from build123d import *

# Parameters (mm, degrees)
SKETCH1_W           = 86.36
SKETCH1_H           = 76.2
SKETCH1_R           = 1.397
BOSS_EXTRUDE1_DEPTH = 2
SKETCH2_W           = 15.24
SKETCH2_H           = 2.54
BOSS_EXTRUDE2_DEPTH = 40


with BuildPart() as part:
    # Sketch1 → Boss-Extrude1 (new body)
    with BuildSketch(Plane(origin=(0, 0, 0), x_dir=(1, 0, 0), z_dir=(0, 1, 0))):
        Rectangle(SKETCH1_W, SKETCH1_H)
        with Locations((-39.37, 34.29)):
            Circle(SKETCH1_R, mode=Mode.SUBTRACT)
        with Locations((39.37, -34.29)):
            Circle(SKETCH1_R, mode=Mode.SUBTRACT)
        with Locations((-39.37, -34.29)):
            Circle(SKETCH1_R, mode=Mode.SUBTRACT)
        with Locations((39.37, 34.29)):
            Circle(SKETCH1_R, mode=Mode.SUBTRACT)
    extrude(amount=BOSS_EXTRUDE1_DEPTH)

    # Sketch2 → Boss-Extrude2 (add)
    with BuildSketch(Plane(origin=(0, 2, 0), x_dir=(1, 0, 0), z_dir=(0, 1, 0))):
        with Locations((-16.51, 2.54)):
            Rectangle(SKETCH2_W, SKETCH2_H)
    extrude(amount=BOSS_EXTRUDE2_DEPTH)


solid = part.part
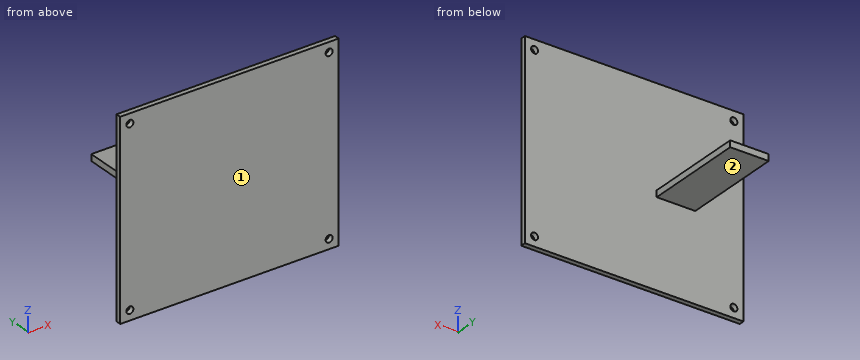
Check sheet for the modelled part. Datum: model origin and axes. Units: mm. Face numbers are marked on the shaded views. A direction names the side the tool comes from. Coordinates: 2 decimals unless noted, no trailing zeros. Loops run counter-clockwise (first coordinate to the right, second up) from the corner with the lowest first, then second, coordinate; pieces in that order, holes last. Notation, with made-up numbers: (-34, 52.5) -> (17, 52.5) arc R27 cw to (17, 86.5) -> close; hole circle Ø6 at (57, 51.25). An arc over 180 degrees is marked (long way). Write item = value, one per line. Start each with the question number.
1. Depth check by flat-ended pin: P1, Ø7.5, axis at x = -19, y = 18.5, coming from the -Z side; P2, Ø1.7, axis at x = -39.37, z = 34.29, coming from the +Y side; P3, Ø3, axis at x = 20, z = -18, coming from the +Y side; P4, Ø12, axis at x = -16, y = 26.5, coming from the +Z side. Enter the tip coordinate at first touch or a pass-through.
2. Section check D-D on y = 33. Record the cut outline in (x, z).
3. Section check C-C on x = -16. Record the cut outline in (y, z), then the cut area to 3 significant figures.
4. Material ranges on line 1 (Z direction, x = -39.37, y = 0.55); line 2 (X direction, y = 1.1, z = 34.29); line 3 (Z direction, x = -39, y = 1), recorded low to high.
5. Section check A-A on z = 34.29. Record the cut outline in (x, y), then the cut area to 3 significant figures.
6. Tool access check on the marked faces 1 and 2. Record the directions out of +Z, -Z, +X, -X, +Y, -Y that give a thin tool (end or side, any length) a straight path to the whole face; none if there is none.
7. Section check B-B on x = 39.37. Record the cut outline in (y, z).
Responses:
q1.P1 = -3.81
q1.P2 = through
q1.P3 = 2
q1.P4 = -1.27
q2.outline = (-24.13, -3.81) -> (-8.89, -3.81) -> (-8.89, -1.27) -> (-24.13, -1.27) -> close
q3.outline = (0, -38.1) -> (2, -38.1) -> (2, -3.81) -> (42, -3.81) -> (42, -1.27) -> (2, -1.27) -> (2, 38.1) -> (0, 38.1) -> close
q3.area = 254 mm2
q4.line_1 = -38.1 to -35.69, -32.89 to 32.89, 35.69 to 38.1
q4.line_2 = -43.18 to -40.77, -37.97 to 37.97, 40.77 to 43.18
q4.line_3 = -38.1 to -35.64, -32.94 to 32.94, 35.64 to 38.1
q5.outline = (-43.18, 0) -> (-40.77, 0) -> (-40.77, 2) -> (-43.18, 2) -> close; (-37.97, 0) -> (37.97, 0) -> (37.97, 2) -> (-37.97, 2) -> close; (40.77, 0) -> (43.18, 0) -> (43.18, 2) -> (40.77, 2) -> close
q5.area = 162 mm2
q6.face_1 = +Z, -Z, +X, -X, -Y
q6.face_2 = -Z, +X, -X, +Y
q7.outline = (0, -38.1) -> (2, -38.1) -> (2, -35.69) -> (0, -35.69) -> close; (0, -32.89) -> (2, -32.89) -> (2, 32.89) -> (0, 32.89) -> close; (0, 35.69) -> (2, 35.69) -> (2, 38.1) -> (0, 38.1) -> close
